from build123d import *

# Parameters (mm, degrees)
SKETCH_W          = 101
SKETCH_H          = 25.4
PAD_DEPTH         = 3.5
SKETCH001_W       = 12.5
SKETCH001_H       = 7
POCKET_DEPTH      = 3.501
POCKET_DEPTH_BACK = 0.001
FILLET_R          = 0.5


with BuildPart() as part:
    # Sketch → Pad (new body)
    with BuildSketch(Plane.XZ):
        Rectangle(SKETCH_W, SKETCH_H)
    extrude(amount=PAD_DEPTH)

    # Sketch001 (on DatumPlane) → Pocket (cut, two sides)
    with BuildSketch(Plane.XZ.offset(3.5)) as pocket_sk:
        Polygon((-48, 5.8), (-48, 0.8), (-26, 0.8), (-26, 0.3), (-17.5, 0.3), (-17.5, -10.7), (17.5, -10.7), (17.5, 0.3), (26, 0.3), (26, 0.8), (48, 0.8), (48, 5.8), (26, 5.8), (26, 6.3), (17.5, 6.3), (17.5, 8.8), (-17.5, 8.8), (-17.5, 6.3), (-26, 6.3), (-26, 5.8), align=None)
        with Locations((30, -6.2)):
            Rectangle(SKETCH001_W, SKETCH001_H)
    extrude(amount=-POCKET_DEPTH, mode=Mode.SUBTRACT)
    extrude(pocket_sk.sketch, amount=POCKET_DEPTH_BACK, mode=Mode.SUBTRACT)

    # Fillet
    fillet_edges = [part.edges().sort_by_distance(p)[0] for p in [
        (23.75, -3.5, -6.2),
        (23.75, -1.75, -9.7),
        (23.75, 0, -6.2),
        (23.75, -1.75, -2.7),
        (30, -3.5, -9.7),
        (36.25, -1.75, -9.7),
        (30, 0, -9.7),
        (30, -3.5, -2.7),
        (30, 0, -2.7),
        (36.25, -1.75, -2.7),
        (36.25, -3.5, -6.2),
        (36.25, 0, -6.2),
    ]]
    fillet(fillet_edges, radius=FILLET_R)


solid = part.part
Work out the finished part from the listing and answer in its coordinate system (mm). A direction names the side the tool comes from. Give positions to 0.01 mm unless a question says otherwise; leave off trailing zeros. Loops run counter-clockwise (first coordinate to the right, second up) from the corner with the lowest first, then second, coordinate; pieces in that order, holes last. Notation, with made-up numbers: (58.25, -28) - (87.25, -28) arc R29 ccw to (87.25, 11) - close; hole circle Ø4 at (73, 25). An arc over 180 degrees is marked (long way). Answer in a Markdown table with one row per item. Add a question column.
Q1. Consider line 1 along X through (y, z) = (-1.3, -5); line 2 along Z through (x, y) = (8.5, -2.15); line 3 along X through (y, z) = (-0.45, 3.5). Determine where each line is inside the solid, lowest interval first.
Q2. Determine the mould class of faces 3 (the flat face through (-1, 0, -11)), 4 (the flat face through (17.5, -2, 8)), 5 (the flat face through (-50.5, -2, 0)) for opening direction X: released by +X, released by -X, zero draft, split by the parting line, or undercut.
Q3. A tool of negligible diameter and unlimited length cuts with its end or side. For faces 1 (the flat face through (22, -2, 6.3)), 2 (the flat face through (-1, -2, 12.7)), from which of +Z, -Z, +X, -X, +Y, -Y can it reach the whole face along a straight path? Write none if from no direction.
Q4. The part is cut by section B-B (x = 1.5). Determine the outline of the cut face in (y, z).
Q5. The part is cut by section A-A (z = -7). Determine the outline of the cut face in (x, y), and give its area (3 significant figures).
Q6. The part is cut by section C-C (y = -1.15). State how many separate pieces and enclosed holes the cut face has, and give its area (3 significant figures).
Q7. The part is cut by section D-D (z = 3.75). Determine the outline of the cut face in (x, y), and give its area (3 significant figures).
Solution:
| question | item | result |
|---|---|---|
| 1 | line 1 | x = -50.5 to -17.5, 17.5 to 23.75, 36.25 to 50.5 |
| 1 | line 2 | z = -12.7 to -10.7, 8.8 to 12.7 |
| 1 | line 3 | x = -50.5 to -48, 48 to 50.5 |
| 2 | face 3 | zero draft |
| 2 | face 4 | undercut |
| 2 | face 5 | released by -X |
| 3 | face 1 | +Y, -Y |
| 3 | face 2 | +Z, +X, -X, +Y, -Y |
| 4 | outline | (-3.5, -12.7) - (0, -12.7) - (0, -10.7) - (-3.5, -10.7) - close; (-3.5, 8.8) - (0, 8.8) - (0, 12.7) - (-3.5, 12.7) - close |
| 5 | outline | (-50.5, -3.5) - (-17.5, -3.5) - (-17.5, 0) - (-50.5, 0) - close; (17.5, -3.5) - (23.25, -3.5) arc R0.5 ccw to (23.75, -3) - (23.75, -0.5) arc R0.5 ccw to (23.25, 0) - (17.5, 0) - close; (36.25, -3) arc R0.5 ccw to (36.75, -3.5) - (50.5, -3.5) - (50.5, 0) - (36.75, 0) arc R0.5 ccw to (36.25, -0.5) - close |
| 5 | area | 187 mm² |
| 6 | separate pieces | 1 |
| 6 | enclosed holes | 2 |
| 6 | area | 1,470 mm² |
| 7 | outline | (-50.5, -3.5) - (-48, -3.5) - (-48, 0) - (-50.5, 0) - close; (48, -3.5) - (50.5, -3.5) - (50.5, 0) - (48, 0) - close |
| 7 | area | 17.5 mm² |
